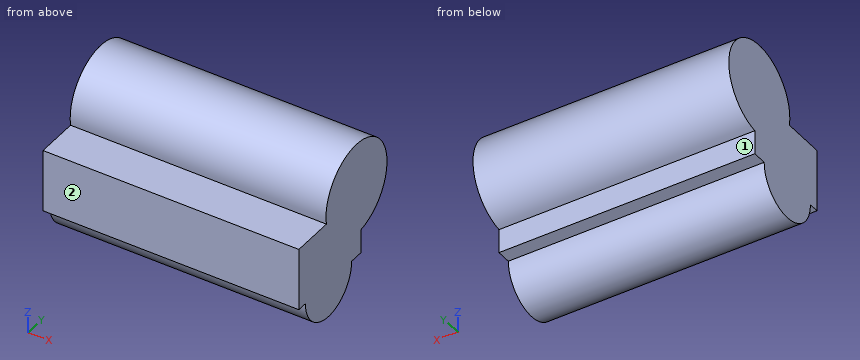
Autodesk Inventor part; units mm, degrees
ref_plane "YZ Plane" through (0, 0, 0) normal (1, 0, 0) x (0, 1, 0)
ref_plane "XZ Plane" through (0, 0, 0) normal (0, 1, 0) x (-1, 0, 0)
ref_plane "XY Plane" through (0, 0, 0) normal (0, 0, 1) x (1, 0, 0)
sketch "Sketch1" plane through (0, 0, 0) normal (1, 0, 0) x (0, 1, 0)
  circle A0 centre (5.3535, -5.8605) radius 7.071
  circle A1 centre (13.9111, 8.1317) radius 9.3306
  line L0 (-3.7313, 6.6311) -> (15.29, 6.6311)
  line L1 (15.29, 6.6311) -> (15.29, -5.8605)
  line L2 (15.29, -5.8605) -> (-3.7313, -5.8605)
  line L3 (-3.7313, -5.8605) -> (-3.7313, 6.6311)
  point P0 (0, 0)
extrude "Extrusion1" add sketch "Sketch1" along normal blind 50.8
properties part number "test"
Verification items for the finished model (mm, model axes). Face numbers are marked on the shaded views. A direction names the side the tool comes from. Give positions to 0.01 mm unless a question says otherwise; leave off trailing zeros. Loops run counter-clockwise (first coordinate to the right, second up) from the corner with the lowest first, then second, coordinate; pieces in that order, holes last.
1) Sectioned sample at B-B, the plane y = 8.75. Enter the section's corners in (x, z).
2) Depth check by flat-ended pin: pin 1 Ø10 at (x, y) = (32, 15) entering from +Z; pin 2 Ø9.5 at (x, y) = (34.5, 2.5) entering from +Z; pin 3 Ø2.5 at (x, z) = (34, -4) entering from +Y; pin 4 Ø1.4 at (x, y) = (13, 14.5) entering from -Z. Enter the tip coordinate at first touch or a pass-through.
3) Sectioned sample at C-C, the plane z = -0.5. Enter the section's corners in (x, y), then the cut area to 3 significant figures.
4) Set-up check for the marked faces 1 and 2: record each of +Z, -Z, +X, -X, +Y, -Y from which the full face is reachable in a straight line by a thin tool's end or side.
5) Thickness scan on line 1 along Y through (x, z) = (12, -5.5); line 2 along Y through (x, z) = (25.5, -6); line 3 along Z through (x, y) = (4, 8.25). Record the ranges inside material, lowest first.
6) Sectioned sample at A-A, the plane x = 24. Enter the section's corners in (y, z).
Answers:
1. outline: (0, -12.06) - (50.8, -12.06) - (50.8, 15.9) - (0, 15.9) - close
2. pin 1: stops at z = 17.46
2. pin 2: stops at z = 14.67
2. pin 3: stops at y = 15.29
2. pin 4: stops at z = -5.86
3. outline: (0, -3.73) - (50.8, -3.73) - (50.8, 17.45) - (0, 17.45) - close
3. area: 1,080 mm2
4. face 1: -Z, +X, -X, +Y
4. face 2: +Z, -Z, +X, -X, -Y
5. line 1: y = -3.73 to 15.29
5. line 2: y = -1.72 to 12.42
5. line 3: z = -12.31 to 15.55
6. outline: (-3.73, -5.86) - (-1.72, -5.86) arc R7.07 ccw to (12.42, -5.86) - (15.29, -5.86) - (15.29, -1.1) arc R9.33 ccw (long way) to (4.7, 6.63) - (-3.73, 6.63) - close
